```python
from build123d import *

# Parameters (mm, degrees)
F2_R     = 3.3
F3_DEPTH = 64.001
F4_R     = 5.5
F5_DEPTH = 6.1
F6_R     = 1
F7_SIZE2 = 1
F7_SIZE  = 1
F8_SIZE  = 1


with BuildPart() as f1:
    # F0 (on Front) → F1 (revolve)
    with BuildSketch(Plane.XZ):
        Polygon((15, 64), (15, 0), (37, 0), (37, 10), (22.5, 10), (22.5, 64), align=None)
    revolve(axis=Axis((0, 0, 43.789597), (0, 0, 1)))

    # F2 (on face) → F3 (cut, through all)
    with BuildSketch(Plane(origin=(0, 0, 0), x_dir=(1, 0, 0), z_dir=(0, 0, -1))):
        with Locations((0, 30)):
            Circle(F2_R)
        with Locations((-30, 0)):
            Circle(F2_R)
        with Locations((0, -30)):
            Circle(F2_R)
        with Locations((30, 0)):
            Circle(F2_R)
    extrude(amount=-F3_DEPTH, mode=Mode.SUBTRACT)

    # F4 (on face) → F5 (cut)
    with BuildSketch(Plane(origin=(0, 0, 0), x_dir=(1, 0, 0), z_dir=(0, 0, -1))):
        with Locations((0, 30)):
            Circle(F4_R)
        with Locations((30, 0)):
            Circle(F4_R)
        with Locations((-30, 0)):
            Circle(F4_R)
        with Locations((0, -30)):
            Circle(F4_R)
    extrude(amount=-F5_DEPTH, mode=Mode.SUBTRACT)

    # F6
    f6_edges = [f1.edges().sort_by_distance(p)[0] for p in [
        (-22.5, 0, 10),
    ]]
    fillet(f6_edges, radius=F6_R)

    # F7
    f7_edges = [f1.edges().sort_by_distance(p)[0] for p in [
        (-15, 0, 0),
    ]]
    chamfer(f7_edges, length=F7_SIZE, length2=F7_SIZE2)

    # F8
    f8_edges = [f1.edges().sort_by_distance(p)[0] for p in [
        (-15, 0, 64),
    ]]
    chamfer(f8_edges, length=F8_SIZE)


solid = f1.part
```
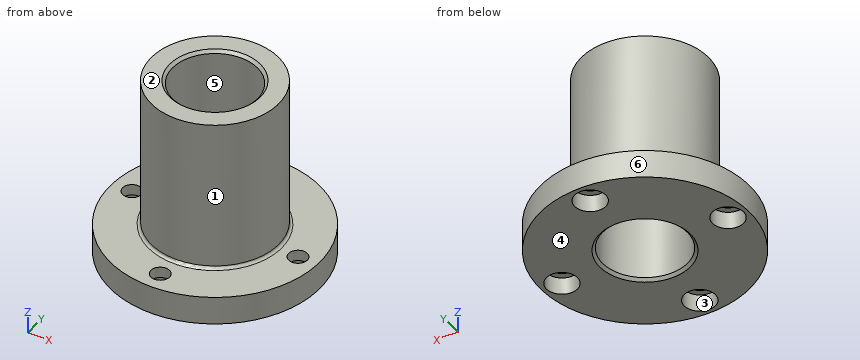
For this review, take the finished solid that the model builds, in its own axes (mm). Face numbers are marked on the shaded views. A direction names the side the tool comes from. Give positions to 0.01 mm unless a question says otherwise; leave off trailing zeros. Loops run counter-clockwise (first coordinate to the right, second up) from the corner with the lowest first, then second, coordinate; pieces in that order, holes last. Notation, with made-up numbers: M -10.5,-36.5 L 24.5,-36.5 A27 cw 24.5,0.5 Z; hole C 84,17.25 d9. An arc over 180 degrees is marked long. One line per item, written item: value. Start each with the question number.
Q1. Machinability: for the marked faces 1, 2 and 3, which of the approach directions +Z, -Z, +X, -X, +Y, -Y give a long, thin tool a straight path to every point of the face, cutting with its end or side? Answer none if there is none.
Q2. For L1, parallel to Y at x = 0, z = 7; L2, parallel to Y at x = 0, z = 1; L3, parallel to Y at x = 0, z = 15.5, list the stretches that pass through material, from the lowest coordinate up.
Q3. Add section C-C (x = 30). Give the boundary of the cut face in (y, z).
Q4. Add section D-D (z = 23). Give the boundary of the cut face in (x, y).
Q5. Draft analysis for pull direction Y (two halves, no side actions). For the marked faces 4, 5 and 6, state which applies: released by +Y, released by -Y, zero draft, split by the parting line, or undercut.
Q6. Clearance check with flat-ended pins moving along their axes: pin 1 Ø6.5 at (x, y) = (30, 0) entering from -Z; pin 2 Ø7.5 at (x, y) = (-30, 0) entering from -Z; pin 3 Ø8.5 at (x, y) = (0, -30) entering from +Z; pin 4 Ø3 at (x, z) = (-12, 40.5) entering from -Y. State where each tip first meets the part, or that it passes through.
Q7. Add section A-A (x = 0). Count the separate pieces of the cut face and the enclosed holes in it, and give its area (3 significant figures).
Reply:
1. face 1: +Z
1. face 2: +Z, +X, -X, +Y, -Y
1. face 3: -Z
2. L1: -37 to -33.3, -26.7 to -15, 15 to 26.7, 33.3 to 37
2. L2: -37 to -35.5, -24.5 to -15, 15 to 24.5, 35.5 to 37
2. L3: -22.5 to -15, 15 to 22.5
3. outline: M -21.66,0 L -5.5,0 L -5.5,6.1 L -3.3,6.1 L -3.3,10 L -21.66,10 Z; M 3.3,6.1 L 5.5,6.1 L 5.5,0 L 21.66,0 L 21.66,10 L 3.3,10 Z
4. outline: C 0,0 d45; hole C 0,0 d30
5. face 4: zero draft
5. face 5: undercut
5. face 6: split by the parting line
6. pin 1: through
6. pin 2: z = 6.1
6. pin 3: z = 10
6. pin 4: y = -19.9
7. separate pieces: 4
7. enclosed holes: 0
7. area: 1,060 mm²
